Here's how the part is built. I have some questions about the finished solid (model axes, mm). Coordinates: 2 decimals unless noted, no trailing zeros. Order: outer loops, then holes, each group sorted by start corner. A loop starts at its lowest first (then second) coordinate and runs counter-clockwise, first axis right, second up. Notation, with made-up numbers: M 84.5,72.25 L 89.5,72.25 A13 ccw 89.5,93.25 Z; hole C -2.5,64 d5. An arc over 180 degrees is marked long. One line per question, with ' | ' between items. Start each with the question number.
```python
from build123d import *

# Parameters (mm, degrees)
SKETCH2_W           = 170
SKETCH2_H           = 30
BOSS_EXTRUDE2_DEPTH = 6
BOSS_EXTRUDE4_DEPTH = 6
CHAMFER1_SIZE       = 2
HOLE6_D             = 4.5
HOLE4_D             = 4.5
HOLE7_D             = 15


with BuildPart() as part:
    # Sketch2 → Boss-Extrude2 (new body)
    with BuildSketch(Plane(origin=(0, 0, 0), x_dir=(0, 1, 0), z_dir=(0, 0, 1))):
        Rectangle(SKETCH2_W, SKETCH2_H)
    extrude(amount=BOSS_EXTRUDE2_DEPTH)

    # Sketch8 → Boss-Extrude4 (add)
    with BuildSketch(Plane.XY.offset(6)):
        Polygon((-30, -110.980762114), (-15, -136.961524227), (15, -136.961524227), (30, -110.980762114), (15, -85), (-15, -85), align=None)
    extrude(amount=-BOSS_EXTRUDE4_DEPTH)

    # Chamfer1
    chamfer1_edges = [part.edges().sort_by_distance(p)[0] for p in [
        (-22.5, -97.990381057, 0),
        (22.5, -97.990381057, 0),
        (22.5, -123.97114317, 0),
        (0, -136.961524227, 0),
        (-22.5, -123.97114317, 0),
        (-22.5, -97.990381057, 6),
        (15, 0, 6),
        (-22.5, -123.97114317, 6),
        (0, -136.961524227, 6),
        (22.5, -123.97114317, 6),
        (22.5, -97.990381057, 6),
        (0, 85, 6),
        (15, 0, 0),
        (-15, 0, 0),
        (0, 85, 0),
        (-15, 0, 6),
    ]]
    chamfer(chamfer1_edges, length=CHAMFER1_SIZE)

    # Hole6 (through all)
    with Locations(Plane(origin=(0, 0, 0), x_dir=(-1, 0, 0), z_dir=(0, 0, -1))):
        with Locations((8, -116.961524227), (-8, -116.961524227), (-8, -100.961524227), (8, -100.961524227)):
            Hole(HOLE6_D / 2)

    # Hole4 (through all)
    with Locations(Plane.XY.offset(6)):
        with Locations((-5, 68), (5, 68), (5, 78), (-5, 78)):
            Hole(HOLE4_D / 2)

    # Hole7 (through all)
    with Locations(Plane(origin=(0, -108.961524227, 6), x_dir=(1, 0, 0), z_dir=(0, 0, 1))):
        with Locations((0, 0)):
            Hole(HOLE7_D / 2)


solid = part.part
```
1. Will these pins go through, and if not, where does the flat tip stop? pin 1 (3 mm diameter, centred on y = -96, z = 1.5, fed in from -X); pin 2 (3 mm diameter, centred on y = -69, z = 1.5, fed in from -X); pin 3 (10 mm diameter, centred on x = 23, y = -22.5, fed in from +Z); pin 4 (1.6 mm diameter, centred on y = 5, z = 3, fed in from +X).
2. Imagine slicing it at B-B (x = 0). List the corners of the cut face in (y, z) for me, then the cut area to 3 significant figures.
3. Imagine slicing it at A-A (y = 78). List the corners of the cut face in (x, z) for me, then the cut area to 3 significant figures.
4. Imagine slicing it at C-C (y = -64.5). List the corners of the cut face in (x, z) for me, then the cut area to 3 significant figures.
5. I need wall thicknesses on line 1 (Y direction, x = 8, z = 2.9); line 2 (Y direction, x = 5, z = 4.5); line 3 (Y direction, x = 8, z = 1.5). Which ranges of each line are inside material? Lowest first, please.
6. We'd pull the mould along Y, two halves only. Please class faces 1 (the face through (22.605, -98.172, 3.014)), 2 (the face through (-21.73, -123.28, 5.01)), 3 (the face through (0.976, -101.525, 2.958)): released by +Y, released by -Y, zero draft, split by the parting line, or undercut.
7. Imagine slicing it at D-D (z = 3). Count the separate pieces of the cut face and the enclosed holes in it, then the cut area to 3 significant figures.
Entries:
1) pin 1: x = -22.17 | pin 2: x = -15 | pin 3: through | pin 4: x = 15
2) outline: M -136.96,2 L -134.96,0 L -116.46,0 L -116.46,6 L -134.96,6 L -136.96,4 Z; M -101.46,0 L 83,0 L 85,2 L 85,4 L 83,6 L -101.46,6 Z | area: 1,230 mm²
3) outline: M -15,2 L -13,0 L -7.25,0 L -7.25,6 L -13,6 L -15,4 Z; M -2.75,0 L 2.75,0 L 2.75,6 L -2.75,6 Z; M 7.25,0 L 13,0 L 15,2 L 15,4 L 13,6 L 7.25,6 Z | area: 118 mm²
4) outline: M -15,2 L -13,0 L 13,0 L 15,2 L 15,4 L 13,6 L -13,6 L -15,4 Z | area: 172 mm²
5) line 1: -136.96 to -119.21, -114.71 to -103.21, -98.71 to 85 | line 2: -136.46 to -114.55, -103.37 to 65.75, 70.25 to 75.75, 80.25 to 84.5 | line 3: -136.46 to -119.21, -114.71 to -103.21, -98.71 to 84.5
6) face 1: released by +Y | face 2: released by -Y | face 3: undercut
7) separate pieces: 1 | enclosed holes: 9 | area: 7,130 mm²
